from build123d import *

# Parameters (mm, degrees)
SKETCH_1_W          = 143
SKETCH_1_H          = 125
EXTRUDE_1_DEPTH     = 2
FILLET_1_R          = 3
SKETCH_2_R          = 6
CUT_EXTRUDE_1_DEPTH = 10
SKETCH_3_R          = 1.2
CUT_EXTRUDE_2_DEPTH = 10


with BuildPart() as part:
    # 草图1 → 凸台-拉伸1 (new body)
    with BuildSketch(Plane.XY):
        Rectangle(SKETCH_1_W, SKETCH_1_H)
    extrude(amount=EXTRUDE_1_DEPTH)

    # 圆角1
    fillet_1_edges = [part.edges().sort_by_distance(p)[0] for p in [
        (-71.5, 62.5, 1),
        (71.5, 62.5, 1),
        (71.5, -62.5, 1),
        (-71.5, -62.5, 1),
    ]]
    fillet(fillet_1_edges, radius=FILLET_1_R)

    # 草图2 → 切除-拉伸1 (cut)
    with BuildSketch(Plane(origin=(0, 0, 0), x_dir=(-1, 0, 0), z_dir=(0, 0, -1))):
        Circle(SKETCH_2_R)
        with Locations((18, 0)):
            Circle(SKETCH_2_R)
        with Locations((36, 0)):
            Circle(SKETCH_2_R)
        with Locations((54, 0)):
            Circle(SKETCH_2_R)
        with Locations(Location((-54, 0, 0), (0, 0, 180))):
            Circle(SKETCH_2_R)
        with Locations(Location((-36, 0, 0), (0, 0, 180))):
            Circle(SKETCH_2_R)
        with Locations(Location((-18, 0, 0), (0, 0, 180))):
            Circle(SKETCH_2_R)
        with Locations((0, 16)):
            Circle(SKETCH_2_R)
        with Locations((18, 16)):
            Circle(SKETCH_2_R)
        with Locations((36, 16)):
            Circle(SKETCH_2_R)
        with Locations((54, 16)):
            Circle(SKETCH_2_R)
        with Locations(Location((-54, 16, 0), (0, 0, 180))):
            Circle(SKETCH_2_R)
        with Locations(Location((-36, 16, 0), (0, 0, 180))):
            Circle(SKETCH_2_R)
        with Locations(Location((-18, 16, 0), (0, 0, 180))):
            Circle(SKETCH_2_R)
        with Locations((0, 32)):
            Circle(SKETCH_2_R)
        with Locations((18, 32)):
            Circle(SKETCH_2_R)
        with Locations((36, 32)):
            Circle(SKETCH_2_R)
        with Locations((54, 32)):
            Circle(SKETCH_2_R)
        with Locations(Location((-54, 32, 0), (0, 0, 180))):
            Circle(SKETCH_2_R)
        with Locations(Location((-36, 32, 0), (0, 0, 180))):
            Circle(SKETCH_2_R)
        with Locations(Location((-18, 32, 0), (0, 0, 180))):
            Circle(SKETCH_2_R)
        with Locations((0, 48)):
            Circle(SKETCH_2_R)
        with Locations((18, 48)):
            Circle(SKETCH_2_R)
        with Locations((36, 48)):
            Circle(SKETCH_2_R)
        with Locations((54, 48)):
            Circle(SKETCH_2_R)
        with Locations(Location((-54, 48, 0), (0, 0, 180))):
            Circle(SKETCH_2_R)
        with Locations(Location((-36, 48, 0), (0, 0, 180))):
            Circle(SKETCH_2_R)
        with Locations(Location((-18, 48, 0), (0, 0, 180))):
            Circle(SKETCH_2_R)
        with Locations((0, -16)):
            Circle(SKETCH_2_R)
        with Locations((18, -16)):
            Circle(SKETCH_2_R)
        with Locations((36, -16)):
            Circle(SKETCH_2_R)
        with Locations((54, -16)):
            Circle(SKETCH_2_R)
        with Locations(Location((-54, -16, 0), (0, 0, 180))):
            Circle(SKETCH_2_R)
        with Locations(Location((-36, -16, 0), (0, 0, 180))):
            Circle(SKETCH_2_R)
        with Locations(Location((-18, -16, 0), (0, 0, 180))):
            Circle(SKETCH_2_R)
        with Locations((0, -32)):
            Circle(SKETCH_2_R)
        with Locations((18, -32)):
            Circle(SKETCH_2_R)
        with Locations((36, -32)):
            Circle(SKETCH_2_R)
        with Locations((54, -32)):
            Circle(SKETCH_2_R)
        with Locations(Location((-54, -32, 0), (0, 0, 180))):
            Circle(SKETCH_2_R)
        with Locations(Location((-36, -32, 0), (0, 0, 180))):
            Circle(SKETCH_2_R)
        with Locations(Location((-18, -32, 0), (0, 0, 180))):
            Circle(SKETCH_2_R)
        with Locations((0, -48)):
            Circle(SKETCH_2_R)
        with Locations((18, -48)):
            Circle(SKETCH_2_R)
        with Locations((36, -48)):
            Circle(SKETCH_2_R)
        with Locations((54, -48)):
            Circle(SKETCH_2_R)
        with Locations(Location((-54, -48, 0), (0, 0, 180))):
            Circle(SKETCH_2_R)
        with Locations(Location((-36, -48, 0), (0, 0, 180))):
            Circle(SKETCH_2_R)
        with Locations(Location((-18, -48, 0), (0, 0, 180))):
            Circle(SKETCH_2_R)
    extrude(amount=-CUT_EXTRUDE_1_DEPTH, mode=Mode.SUBTRACT)

    # 草图3 → 切除-拉伸2 (cut)
    with BuildSketch(Plane.XY.offset(2)):
        with Locations((-68.5, 37.12550176)):
            Circle(SKETCH_3_R)
        with Locations((-68.5, 17.12550176)):
            Circle(SKETCH_3_R)
        with Locations((68.5, 17.12550176)):
            Circle(SKETCH_3_R)
        with Locations((68.5, 37.12550176)):
            Circle(SKETCH_3_R)
    extrude(amount=-CUT_EXTRUDE_2_DEPTH, mode=Mode.SUBTRACT)


solid = part.part
Work out the finished part from the listing and answer in its coordinate system (mm). Coordinates: 2 decimals unless noted, no trailing zeros. Use one line per item in the form item = value. Start each with the question number.
1. A straight line is drawn through the part: probe 1 along Y at (x, z) = (-68.5, 0.8). Find the intervals that lie inside material, in ascending order. Write a range as from..to.
2. The mould has two halves that part along X. Classify faces 1 (the face through (-48, 16, 1)), 2 (the face through (-70.64, 61.6, 1.01)), 3 (the face through (31, -27, 2)): released by +X, released by -X, zero draft, split by the parting line, or undercut.
3. The part is cut by section A-A (y = -48). Give the number of separate pieces and of enclosed holes in the cut face, plus the area to 3 significant figures.
Evaluation:
q1.probe_1 = -62.5..15.93, 18.33..35.93, 38.33..62.5
q2.face_1 = undercut
q2.face_2 = released by -X
q2.face_3 = zero draft
q3.separate_pieces = 8
q3.enclosed_holes = 0
q3.area = 118 mm^2
